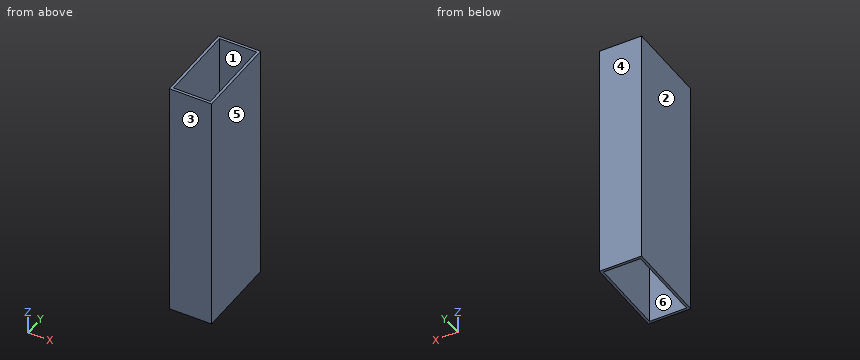
Autodesk Inventor part; units mm, degrees
ref_plane "YZ Plane" through (0, 0, 0) normal (1, 0, 0) x (0, 1, 0)
ref_plane "XZ Plane" through (0, 0, 0) normal (0, 1, 0) x (-1, 0, 0)
ref_plane "XY Plane" through (0, 0, 0) normal (0, 0, 1) x (1, 0, 0)
sketch "Sketch1" plane through (0, 0, 0) normal (0, 0, 1) x (1, 0, 0)
  line L0 (-12.7, -25.4) -> (12.7, -25.4)
  line L1 (12.7, -25.4) -> (12.7, 25.4)
  line L2 (12.7, 25.4) -> (-12.7, 25.4)
  line L3 (-12.7, 25.4) -> (-12.7, -25.4)
  line L4 (-12.7, -25.4) -> (12.7, 25.4) construction
  line L5 (12.7, -25.4) -> (-12.7, 25.4) construction
  line L6 (-11.1125, 23.8125) -> (11.1125, 23.8125)
  line L7 (11.1125, 23.8125) -> (11.1125, -23.8125)
  line L8 (11.1125, -23.8125) -> (-11.1125, -23.8125)
  line L9 (-11.1125, -23.8125) -> (-11.1125, 23.8125)
  point P0 (0, 0)
  dimension "width" = 25.4
  dimension "height" = 50.8
  dimension "thickness" = 1.5875
extrude "Extrusion1" add sketch "Sketch1" along normal mid plane 146.05
properties part number "CL3-007" material "Aluminum 6061"
Geometry: final body of the model. Coordinates: model frame, mm. Face numbers are marked on the shaded views. A direction names the side the tool comes from. Give positions to 0.01 mm unless a question says otherwise; leave off trailing zeros. Write each loop counter-clockwise with the first axis right and the second up, starting at its lowest first coordinate (ties: lowest second). Pieces come first, ordered by that corner, then holes. Notation, with made-up numbers: M 65,25.25 L 73,25.25 A9 cw 73,31.25 Z; hole C 1.5,49.5 d11. An arc over 180 degrees is marked long. Answer in a Markdown table with one row per item. Add a question column.
(1) Section B-B on x = 7.5. Return loops of the section in (y, z) (1 decimal), and give its area (3 significant figures).
(2) Reachability of the marked faces 5 and 6 from +Z, -Z, +X, -X, +Y, -Y: full face, straight path, thin tool, end or side. Return the list, or none.
(3) Ray query, line 1 (X direction, y = 13, z = -42); line 2 (Y direction, x = 7.5, z = -32.5). Return the intervals inside material, ascending.
(4) Mould query, pull axis Y, two halves, no side actions, for the marked faces 1, 2, 3 and 4. Classes: +Y half, -Y half, draft (parallel to the pull), parting line (faces both ways), or undercut.
(5) Section C-C on z = 0. Return loops of the section in (x, y), and give its area (3 significant figures).
(6) Section A-A on y = 8.5. Return loops of the section in (x, z) (1 decimal), and give its area (3 significant figures).
Result set:
| question | item | result |
|---|---|---|
| 1 | outline | M -25.4,-73 L -23.8,-73 L -23.8,73 L -25.4,73 Z; M 23.8,-73 L 25.4,-73 L 25.4,73 L 23.8,73 Z |
| 1 | area | 464 mm^2 |
| 2 | face 5 | +Z, -Z, +X, +Y, -Y |
| 2 | face 6 | +Z, -Z |
| 3 | line 1 | x = -12.7 to -11.11, 11.11 to 12.7 |
| 3 | line 2 | y = -25.4 to -23.81, 23.81 to 25.4 |
| 4 | face 1 | undercut |
| 4 | face 2 | draft |
| 4 | face 3 | -Y half |
| 4 | face 4 | +Y half |
| 5 | outline | M -12.7,-25.4 L 12.7,-25.4 L 12.7,25.4 L -12.7,25.4 Z; hole M -11.11,-23.81 L 11.11,-23.81 L 11.11,23.81 L -11.11,23.81 Z |
| 5 | area | 232 mm^2 |
| 6 | outline | M -12.7,-73 L -11.1,-73 L -11.1,73 L -12.7,73 Z; M 11.1,-73 L 12.7,-73 L 12.7,73 L 11.1,73 Z |
| 6 | area | 464 mm^2 |
